```python
from build123d import *

# Parameters (mm, degrees)
SKETCH1_R      = 5.9563
EXTRUDE1_DEPTH = 3.175
SKETCH2_R      = 2.3876
EXTRUDE2_DEPTH = 11.548816018
CHAMFER1_SIZE  = 0.254


with BuildPart() as part:
    # Sketch1 → Extrude1 (new, symmetric)
    with BuildSketch(Plane.XY):
        Circle(SKETCH1_R)
    extrude(amount=EXTRUDE1_DEPTH, both=True)

    # Sketch2 → Extrude2 (cut, through all)
    with BuildSketch(Plane.XY.offset(3.175)):
        Circle(SKETCH2_R)
    extrude(amount=-EXTRUDE2_DEPTH, mode=Mode.SUBTRACT)

    # Chamfer1
    chamfer1_edges = [part.edges().sort_by_distance(p)[0] for p in [
        (-5.9563, 0, -3.175),
        (-5.9563, 0, 3.175),
    ]]
    chamfer(chamfer1_edges, length=CHAMFER1_SIZE)


solid = part.part
```
Verification items for the finished model (mm, model axes). Give positions to 0.01 mm unless a question says otherwise; leave off trailing zeros. Loops run counter-clockwise (first coordinate to the right, second up) from the corner with the lowest first, then second, coordinate; pieces in that order, holes last.
1. Section check C-C, the plane z = -2.25. Enter the section's corners in (x, y).
2. Section check A-A, the plane y = 0. Enter the section's corners in (x, z) (3 decimals).
3. Go/stop test with flat-tipped pins: pin 1 Ø3 at (y, z) = (-4.5, 0.5) entering from -X; pin 2 Ø1 at (x, z) = (-1.5, -1) entering from -Y. Record where each tip stops, or that it passes through.
4. Mould release check, pull along Y, two halves, no side actions. Record for faces 1 (the flat face through (2.5, -1.2, -3.175)), 2 (the cylindrical face through (-0.52, -2.33, 0.04)), 3 (the cylindrical face through (-4.73, -3.62, 0.04)): released by +Y, released by -Y, zero draft, split by the parting line, or undercut.
5. Thickness scan on line 1 (Y direction, x = 0, z = 0); line 2 (Y direction, x = -0.75, z = 2.25); line 3 (X direction, y = 2.5, z = 2.5). Record the ranges inside material, lowest first.
Geometry says:
1. outline: circle Ø11.91 at (0, 0); hole circle Ø4.78 at (0, 0)
2. outline: (-5.956, -2.921) - (-5.702, -3.175) - (-2.388, -3.175) - (-2.388, 3.175) - (-5.702, 3.175) - (-5.956, 2.921) - close; (2.388, -3.175) - (5.702, -3.175) - (5.956, -2.921) - (5.956, 2.921) - (5.702, 3.175) - (2.388, 3.175) - close
3. pin 1: stops at x = -5.15
3. pin 2: stops at y = -5.87
4. face 1: zero draft
4. face 2: undercut
4. face 3: split by the parting line
5. line 1: y = -5.96 to -2.39, 2.39 to 5.96
5. line 2: y = -5.91 to -2.27, 2.27 to 5.91
5. line 3: x = -5.41 to 5.41
